```python
from build123d import *

# Parameters (mm, degrees)
EXTRUDE_4_DEPTH     = 15
SKETCH_6_W          = 5.43
SKETCH_6_H          = 10.5
CUT_EXTRUDE_2_DEPTH = 15
SKETCH_7_W          = 2.285
SKETCH_7_H          = 10.5
CUT_EXTRUDE_3_DEPTH = 15
SKETCH_8_W          = 20
SKETCH_8_H          = 16
EXTRUDE_5_DEPTH     = 4
SKETCH_9_R          = 1.1
EXTRUDE_6_DEPTH     = 4


with BuildPart() as part:
    # 草图1 → 凸台-拉伸4 (new body)
    with BuildSketch(Plane(origin=(0, 0, 0), x_dir=(1, 0, 0), z_dir=(0, 1, 0))):
        with BuildLine():
            Line((-35.94125392, 35.792894198), (-35.94125392, 20.722894198))
            Line((-35.94125392, 20.722894198), (-27.94125392, 20.722894198))
            ThreePointArc((-27.94125392, 20.722894198), (-26.527040358, 21.308680636), (-25.94125392, 22.722894198))
            Line((-25.94125392, 22.722894198), (-25.94125392, 33.792894198))
            ThreePointArc((-25.94125392, 33.792894198), (-26.527040358, 35.207107761), (-27.94125392, 35.792894198))
            Line((-27.94125392, 35.792894198), (-35.94125392, 35.792894198))
        make_face()
    extrude(amount=EXTRUDE_4_DEPTH)

    # 草图6 → 切除-拉伸2 (cut)
    with BuildSketch(Plane(origin=(0, 15, 0), x_dir=(1, 0, 0), z_dir=(0, 1, 0))):
        with Locations((-30.94125392, 28.257894198)):
            Rectangle(SKETCH_6_W, SKETCH_6_H)
    extrude(amount=-CUT_EXTRUDE_2_DEPTH, mode=Mode.SUBTRACT)

    # 草图7 → 切除-拉伸3 (cut)
    with BuildSketch(Plane(origin=(0, 15, 0), x_dir=(1, 0, 0), z_dir=(0, 1, 0))):
        with Locations((-34.79875392, 28.257894198)):
            Rectangle(SKETCH_7_W, SKETCH_7_H)
    extrude(amount=-CUT_EXTRUDE_3_DEPTH, mode=Mode.SUBTRACT)

    # 草图8 → 凸台-拉伸5 (add)
    with BuildSketch(Plane(origin=(-25.94125392, 0, 0), x_dir=(0, 0, -1), z_dir=(1, 0, 0))):
        with Locations((30.722894198, 7.5)):
            Rectangle(SKETCH_8_W, SKETCH_8_H)
    extrude(amount=EXTRUDE_5_DEPTH)

    # 草图9 → 凸台-拉伸6 (add)
    with BuildSketch(Plane(origin=(-21.94125392, 0, 0), x_dir=(0, 0, -1), z_dir=(1, 0, 0))):
        with Locations((27.722894198, 11.8)):
            Circle(SKETCH_9_R)
        with Locations((27.722894198, 3.2)):
            Circle(SKETCH_9_R)
    extrude(amount=EXTRUDE_6_DEPTH)


solid = part.part
```
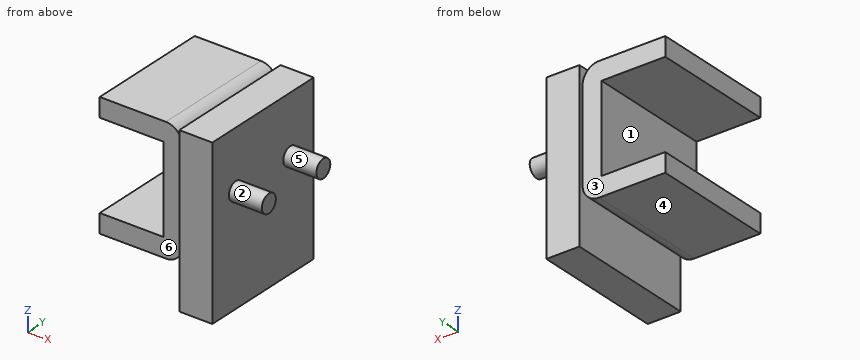
Can you work these out from the model? Positions are in its coordinate system, mm. Face numbers are marked on the shaded views. A direction names the side the tool comes from. Give positions to 0.01 mm unless a question says otherwise; leave off trailing zeros. Write each loop counter-clockwise with the first axis right and the second up, starting at its lowest first coordinate (ties: lowest second). Pieces come first, ordered by that corner, then holes. Notation, with made-up numbers: (78.5, 78) -> (95.5, 78) arc R4 ccw to (95.5, 82) -> close; hole circle Ø8 at (84.5, -2). An arc over 180 degrees is marked (long way). Write item = value, one per line.
(1) Suppose I cut it at A-A on x = -34.5. Write out the boundary of the cut face in (y, z), then the cut area to 4 significant figures.
Worked out:
outline = (0, -35.79) -> (15, -35.79) -> (15, -33.51) -> (0, -33.51) -> close; (0, -23.01) -> (15, -23.01) -> (15, -20.72) -> (0, -20.72) -> close
area = 68.55 mm^2
(2) Thinking about a two-plate mould opening in Y: for the marked faces 4, 5 and 6, which applies, released by +Y, released by -Y, zero draft, split by the parting line, or undercut?
Worked out:
face_4 = zero draft
face_5 = undercut
face_6 = released by -Y
(3) For the marked faces 1, 2 and 3, which set-ups out of +Z, -Z, +X, -X, +Y, -Y let a thin tool reach every point of the face, with its end or its side?
Worked out:
face_1 = -X, +Y, -Y
face_2 = +X
face_3 = +Z, -Z, -X, +Y
(4) Suppose I cut it at B-B on z = -32. Write out the boundary of the cut face in (x, y).
Worked out:
outline = (-28.23, 0) -> (-25.94, 0) -> (-25.94, -0.5) -> (-21.94, -0.5) -> (-21.94, 15.5) -> (-25.94, 15.5) -> (-25.94, 15) -> (-28.23, 15) -> close
(5) Suppose I cut it at D-D on z = -35. Write out the boundary of the cut face in (x, y), then the cut area to 3 significant figures.
Worked out:
outline = (-35.94, 0) -> (-26.35, 0) -> (-26.35, 15) -> (-35.94, 15) -> close; (-25.94, -0.5) -> (-21.94, -0.5) -> (-21.94, 15.5) -> (-25.94, 15.5) -> close
area = 208 mm^2
(6) I'm going to push flat-ended pins straight in: P1, Ø1.5, axis at y = 8, z = -35, coming from the +X side; P2, Ø2.5, axis at x = -33.5, y = 10, coming from the -Z side. Where does each tip first touch, or does it pass through?
Worked out:
P1 = -21.94
P2 = -35.79
(7) I need wall thicknesses on probe 1 along X at (y, z) = (1.25, -33.75); probe 2 along X at (y, z) = (14, -25.5); probe 3 along Z at (x, y) = (-29, 10.5). Which ranges of each line are inside material? Lowest first, please. Write a range as from..to.
Worked out:
probe_1 = -35.94..-21.94
probe_2 = -28.23..-21.94
probe_3 = -35.79..-33.51, -23.01..-20.72
(8) Suppose I cut it at C-C on y = 5.5. Write out the boundary of the cut face in (x, z), then the cut area to 3 significant figures.
Worked out:
outline = (-35.94, -35.79) -> (-27.94, -35.79) arc R2 ccw to (-25.94, -33.79) -> (-25.94, -40.72) -> (-21.94, -40.72) -> (-21.94, -20.72) -> (-25.94, -20.72) -> (-25.94, -22.72) arc R2 ccw to (-27.94, -20.72) -> (-35.94, -20.72) -> (-35.94, -23.01) -> (-28.23, -23.01) -> (-28.23, -33.51) -> (-35.94, -33.51) -> close
area = 148 mm^2
